Drawing for the job (mm, zero at the part's lowest x, y, z). A direction names the side the tool comes from. Coordinates: 2 decimals unless noted, no trailing zeros. Loops run counter-clockwise (first coordinate to the right, second up) from the corner with the lowest first, then second, coordinate; pieces in that order, holes last.
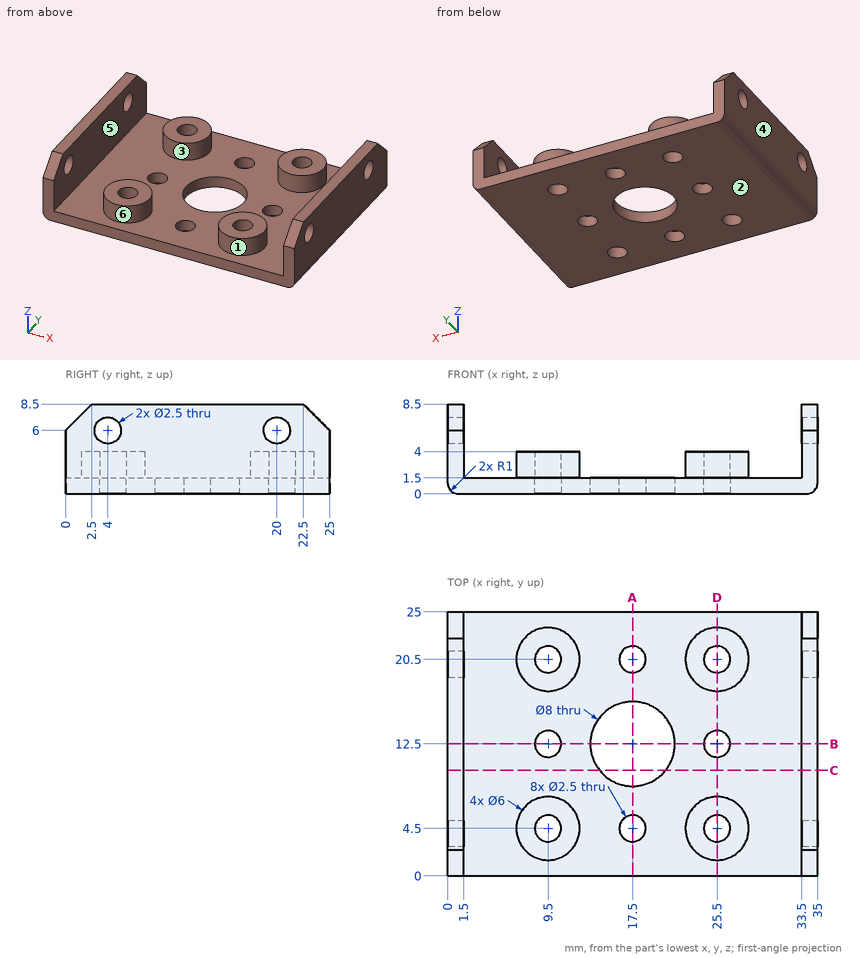
Q1. Mould opens along Y. For the marked faces 1, 2 and 3 say: released by +Y, released by -Y, zero draft, split by the parting line, or undercut.
Q2. Saw through at C-C (y = 10). List the corners of the cut face in (x, z), plus the area to 3 significant figures.
Q3. Saw through at B-B (y = 12.5). List the corners of the cut face in (x, z).
Q4. Tool access for the marked faces 4, 5 and 6: list every direction of +Z, -Z, +X, -X, +Y, -Y with a clear straight run to the whole face (end or side of a thin tool).
Q5. Probe line 1 (Y direction, x = 0.8, z = 6); line 2 (Y direction, x = 25.5, z = 0.55); line 3 (Y direction, x = 9.5, z = 3.4). List the from-to ranges inside material, lowest first.
Q6. Drop flat-ended pins along their axis: P1, Ø5, axis at x = 10.5, y = 19, coming from the +Z side; P2, Ø2, axis at x = 9.5, y = 4.5, coming from the +Z side. Give the stop position or say it passes through.
Q7. Saw through at A-A (x = 17.5). List the corners of the cut face in (y, z), plus the area to 3 significant figures.
Q8. Saw through at D-D (x = 25.5). List the corners of the cut face in (y, z), plus the area to 4 significant figures.
Checked values:
1. face 1: undercut
1. face 2: zero draft
1. face 3: undercut
2. outline: (0, 1) arc R1 ccw to (1, 0) - (14.38, 0) - (14.38, 1.5) - (1.5, 1.5) - (1.5, 8.5) - (0, 8.5) - close; (20.62, 0) - (34, 0) arc R1 ccw to (35, 1) - (35, 8.5) - (33.5, 8.5) - (33.5, 1.5) - (20.62, 1.5) - close
2. area: 63.7 mm2
3. outline: (0, 1) arc R1 ccw to (1, 0) - (8.25, 0) - (8.25, 1.5) - (1.5, 1.5) - (1.5, 8.5) - (0, 8.5) - close; (10.75, 0) - (13.5, 0) - (13.5, 1.5) - (10.75, 1.5) - close; (21.5, 0) - (24.25, 0) - (24.25, 1.5) - (21.5, 1.5) - close; (26.75, 0) - (34, 0) arc R1 ccw to (35, 1) - (35, 8.5) - (33.5, 8.5) - (33.5, 1.5) - (26.75, 1.5) - close
4. face 4: +Z, -Z, -X, +Y, -Y
4. face 5: +Z, +Y, -Y
4. face 6: +Z
5. line 1: y = 0 to 2.75, 5.25 to 18.75, 21.25 to 25
5. line 2: y = 0 to 3.25, 5.75 to 11.25, 13.75 to 19.25, 21.75 to 25
5. line 3: y = 1.5 to 3.25, 5.75 to 7.5, 17.5 to 19.25, 21.75 to 23.5
6. P1: stops at z = 4
6. P2: passes through
7. outline: (0, 0) - (3.25, 0) - (3.25, 1.5) - (0, 1.5) - close; (5.75, 0) - (8.5, 0) - (8.5, 1.5) - (5.75, 1.5) - close; (16.5, 0) - (19.25, 0) - (19.25, 1.5) - (16.5, 1.5) - close; (21.75, 0) - (25, 0) - (25, 1.5) - (21.75, 1.5) - close
7. area: 18.0 mm2
8. outline: (0, 0) - (3.25, 0) - (3.25, 4) - (1.5, 4) - (1.5, 1.5) - (0, 1.5) - close; (5.75, 0) - (11.25, 0) - (11.25, 1.5) - (7.5, 1.5) - (7.5, 4) - (5.75, 4) - close; (13.75, 0) - (19.25, 0) - (19.25, 4) - (17.5, 4) - (17.5, 1.5) - (13.75, 1.5) - close; (21.75, 0) - (25, 0) - (25, 1.5) - (23.5, 1.5) - (23.5, 4) - (21.75, 4) - close
8. area: 43.75 mm2
